```python
from build123d import *

# Parameters (mm, degrees)
F0_W     = 582.2449624538
F0_H     = 123.8665860146
F1_DEPTH = 228.6
F2_W     = 556.8449624538
F2_H     = 203.2
F3_DEPTH = 101.6
F5_DEPTH = 25.4
F7_DEPTH = 25.4


with BuildPart() as f1:
    # F0 (on Front) → F1 (new body)
    with BuildSketch(Plane.XZ):
        with Locations((187.8082603216, -40.8369610086)):
            Rectangle(F0_W, F0_H)
    extrude(amount=F1_DEPTH)

    # F2 (on face) → F3 (cut)
    with BuildSketch(Plane.XY.offset(21.0963319987)):
        with Locations((187.8082603216, -114.3)):
            Rectangle(F2_W, F2_H)
    extrude(amount=-F3_DEPTH, mode=Mode.SUBTRACT)

    # F4 (on face) → F5 (cut)
    with BuildSketch(Plane.YZ.offset(478.9307415485)):
        with BuildLine():
            Line((-81.2571771383, -6.449976629), (-144.7571771383, -6.449976629))
            ThreePointArc((-144.7571771383, -6.449976629), (-149.2473051989, -8.3098485685), (-151.1071771383, -12.799976629))
            Line((-151.1071771383, -12.799976629), (-151.1071771383, -25.499976629))
            ThreePointArc((-151.1071771383, -25.499976629), (-149.2473051989, -29.9901046896), (-144.7571771383, -31.849976629))
            Line((-144.7571771383, -31.849976629), (-81.2571771383, -31.849976629))
            ThreePointArc((-81.2571771383, -31.849976629), (-76.7670490778, -29.9901046896), (-74.9071771383, -25.499976629))
            Line((-74.9071771383, -25.499976629), (-74.9071771383, -12.799976629))
            ThreePointArc((-74.9071771383, -12.799976629), (-76.7670490778, -8.3098485685), (-81.2571771383, -6.449976629))
        make_face()
    extrude(amount=-F5_DEPTH, mode=Mode.SUBTRACT)

    # F6 (on face) → F7 (cut)
    with BuildSketch(Plane(origin=(-103.3142209053, 0, 0), x_dir=(0, -1, 0), z_dir=(-1, 0, 0))):
        with BuildLine():
            Line((147.485794878, -7.8250148058), (83.985794878, -7.8250148058))
            ThreePointArc((83.985794878, -7.8250148058), (79.4956668175, -9.6848867453), (77.635794878, -14.1750148058))
            Line((77.635794878, -14.1750148058), (77.635794878, -26.8750148058))
            ThreePointArc((77.635794878, -26.8750148058), (79.4956668175, -31.3651428663), (83.985794878, -33.2250148058))
            Line((83.985794878, -33.2250148058), (147.485794878, -33.2250148058))
            ThreePointArc((147.485794878, -33.2250148058), (151.9759229385, -31.3651428663), (153.835794878, -26.8750148058))
            Line((153.835794878, -26.8750148058), (153.835794878, -14.1750148058))
            ThreePointArc((153.835794878, -14.1750148058), (151.9759229385, -9.6848867453), (147.485794878, -7.8250148058))
        make_face()
    extrude(amount=-F7_DEPTH, mode=Mode.SUBTRACT)


solid = f1.part
```
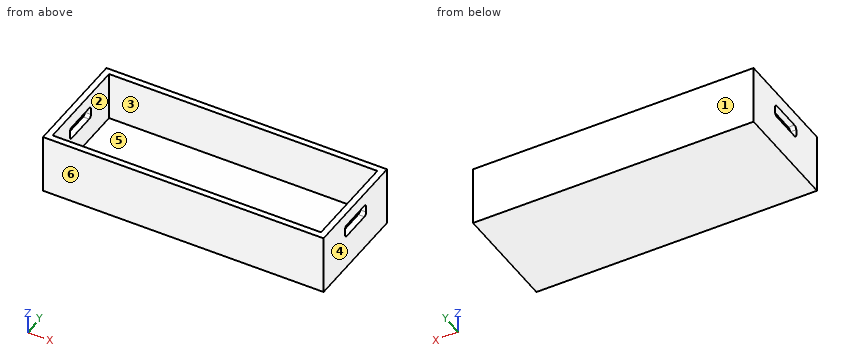
Here's how the part is built. I have some questions about the finished solid (model axes, mm). Face numbers are marked on the shaded views. A direction names the side the tool comes from. Give positions to 0.01 mm unless a question says otherwise; leave off trailing zeros. Loops run counter-clockwise (first coordinate to the right, second up) from the corner with the lowest first, then second, coordinate; pieces in that order, holes last. Notation, with made-up numbers: M 2.25,47 L 43.25,47 A24 cw 43.25,60 Z; hole C -11,35.25 d6. An arc over 180 degrees is marked long. Use one line per item in the form item = value. Start each with the question number.
Q1. Which directions (+Z, -Z, +X, -X, +Y, -Y) give clear straight access to the entire face, cutting with the end or side of a thin tool? Please do the marked faces 5 and 6.
Q2. If we section it at A-A (z = -65): Write out the boundary of the cut face in (x, y), then the cut area to 3 significant figures.
Q3. If we section it at C-C (y = -69.5): Write out the boundary of the cut face in (x, z), then the cut area to 3 significant figures.
Q4. I need wall thicknesses on line 1 along Y through (x, z) = (190, -48.5); line 2 along X through (y, z) = (-157, -21); line 3 along Z through (x, y) = (-18.5, -56.5). Which ranges of each line are inside material? Lowest first, please.
Q5. If we section it at D-D (x = 162): Write out the boundary of the cut face in (y, z), then the cut area to 3 significant figures.
Q6. If we section it at B-B (y = -97.5): Write out the boundary of the cut face in (x, z), then the cut area to 3 significant figures.
Q7. Thinking about a two-plate mould opening in X: for the marked faces 1, 2, 3 and 4, which applies, +X half, -X half, draft (parallel to the pull), parting line (faces both ways), or undercut?
Q8. Will these pins go through, and if not, where does the flat tip stop? pin 1 Ø14 at (x, z) = (475, -18.5) entering from +Y; pin 2 Ø6 at (x, y) = (212, -32) entering from +Z.
Taken from the geometry:
q1.face_5 = +Z
q1.face_6 = +Z, -Z, +X, -X, -Y
q2.outline = M -103.31,-228.6 L 478.93,-228.6 L 478.93,0 L -103.31,0 Z; hole M -90.61,-215.9 L 466.23,-215.9 L 466.23,-12.7 L -90.61,-12.7 Z
q2.area = 20,000 mm^2
q3.outline = M -103.31,-102.77 L 478.93,-102.77 L 478.93,21.1 L 466.23,21.1 L 466.23,-80.5 L -90.61,-80.5 L -90.61,21.1 L -103.31,21.1 Z
q3.area = 15,500 mm^2
q4.line_1 = -228.6 to -215.9, -12.7 to 0
q4.line_2 = -103.31 to -90.61, 466.23 to 478.93
q4.line_3 = -102.77 to -80.5
q5.outline = M -228.6,-102.77 L 0,-102.77 L 0,21.1 L -12.7,21.1 L -12.7,-80.5 L -215.9,-80.5 L -215.9,21.1 L -228.6,21.1 Z
q5.area = 7,670 mm^2
q6.outline = M -103.31,-102.77 L 478.93,-102.77 L 478.93,-31.85 L 466.23,-31.85 L 466.23,-80.5 L -90.61,-80.5 L -90.61,-33.23 L -103.31,-33.23 Z; M -103.31,-7.83 L -90.61,-7.83 L -90.61,21.1 L -103.31,21.1 Z; M 466.23,-6.45 L 478.93,-6.45 L 478.93,21.1 L 466.23,21.1 Z
q6.area = 14,900 mm^2
q7.face_1 = draft
q7.face_2 = undercut
q7.face_3 = undercut
q7.face_4 = +X half
q8.pin_1 = 0
q8.pin_2 = -80.5
